```python
from build123d import *

# Parameters (mm, degrees)
BOSS_EXTRUDE1_DEPTH      = 32.5
BOSS_EXTRUDE1_DEPTH_BACK = 20
BOSS_EXTRUDE2_DEPTH      = 30
BOSS_EXTRUDE4_DEPTH      = 25
SKETCH2_W                = 25
SKETCH2_H                = 25
BOSS_EXTRUDE5_DEPTH      = 30
CUT_EXTRUDE1_DEPTH       = 304.293772711
CUT_EXTRUDE1_DEPTH_BACK  = 304.293772711
SKETCH3_R                = 2.5
SKETCH4_W                = 1
SKETCH4_H                = 30
BOSS_EXTRUDE6_DEPTH      = 15
CUT_EXTRUDE2_DEPTH       = 2
CUT_EXTRUDE2_DEPTH_BACK  = 5
SKETCH5_W                = 24.298824304
SKETCH5_H                = 9.719529722
CUT_EXTRUDE3_REACH       = 305.716
SKETCH6_W                = 258.900724606
SKETCH6_H                = 4.300489871
BOSS_EXTRUDE7_DEPTH      = 20


with BuildPart() as part:
    # Sketch1 → Boss-Extrude1 (new, two sides: drawn at the far end of the back side and taken through both)
    with BuildSketch(Plane(origin=(0, 0, 0), x_dir=(1, 0, 0), z_dir=(0, 1, 0)).offset(-BOSS_EXTRUDE1_DEPTH_BACK)):
        with BuildLine():
            ThreePointArc((-255.2, -34.7), (-259.916681078, 0), (-255.2, 34.7))
            ThreePointArc((-255.2, 34.7), (-294.935777018, 0), (-255.2, -34.7))
        make_face()
    extrude(amount=BOSS_EXTRUDE1_DEPTH + BOSS_EXTRUDE1_DEPTH_BACK)



with BuildPart() as body_2:
    # Sketch1<3> → Boss-Extrude2 (new body)
    with BuildSketch(Plane(origin=(0, 0, 0), x_dir=(1, 0, 0), z_dir=(0, 1, 0))):
        with BuildLine():
            ThreePointArc((0, -37.5), (4.396048304, 0), (0, 37.5))
            Line((0, 37.5), (90, 37.5))
            ThreePointArc((90, 37.5), (127.5, 0), (90, -37.5))
            Line((90, -37.5), (0, -37.5))
        make_face()
    extrude(amount=BOSS_EXTRUDE2_DEPTH)


with BuildPart() as part_1:
    add(part.part)

    add(body_2.part)  # Boss-Extrude4 merges body 2
    # Sketch1<5> → Boss-Extrude4 (add)
    with BuildSketch(Plane(origin=(0, 0, 0), x_dir=(1, 0, 0), z_dir=(0, 1, 0))):
        with BuildLine():
            ThreePointArc((3.700724606, -15), (4.396048304, 0), (3.700724606, 15))
            Line((3.700724606, 15), (-259.04839678, 15))
            ThreePointArc((-259.04839678, 15), (-259.916681078, 0), (-259.04839678, -15))
            Line((-259.04839678, -15), (3.700724606, -15))
        make_face()
    extrude(amount=BOSS_EXTRUDE4_DEPTH)

    # Sketch2 → Boss-Extrude5 (add)
    with BuildSketch(Plane.XZ.offset(20)):
        with Locations((-274.43065957, 0)):
            Rectangle(SKETCH2_W, SKETCH2_H)
    extrude(amount=BOSS_EXTRUDE5_DEPTH)

    # Sketch3 → Cut-Extrude1 (cut, two sides: drawn at the far end of the back side and taken through both)
    with BuildSketch(Plane.XY.offset(12.5).offset(-CUT_EXTRUDE1_DEPTH_BACK)):
        with Locations((-279.13065957, -40)):
            Circle(SKETCH3_R)
    extrude(amount=CUT_EXTRUDE1_DEPTH + CUT_EXTRUDE1_DEPTH_BACK, mode=Mode.SUBTRACT)

    # Sketch4 → Boss-Extrude6 (add)
    with BuildSketch(Plane.XZ):
        with Locations((90, 0)):
            Rectangle(SKETCH4_W, SKETCH4_H)
    extrude(amount=BOSS_EXTRUDE6_DEPTH)

    # Sketch5 → Cut-Extrude2 (cut, two sides: drawn at the far end of the back side and taken through both)
    with BuildSketch(Plane(origin=(90.5, 0, 0), x_dir=(0, 0, -1), z_dir=(1, 0, 0)).offset(-CUT_EXTRUDE2_DEPTH_BACK)):
        with Locations((0, -6.741495989)):
            Rectangle(SKETCH5_W, SKETCH5_H)
    extrude(amount=CUT_EXTRUDE2_DEPTH + CUT_EXTRUDE2_DEPTH_BACK, mode=Mode.SUBTRACT)

    # Cut-Extrude3: up to this face of the body (flat: up to its plane)
    cut_extrude3_end = Plane(part_1.part.faces().sort_by_distance((-127.673836087, 12.5, -15))[0])
    # Sketch6 → Cut-Extrude3 (cut, up to the picked face)
    with BuildSketch(Plane.XY.offset(15), mode=Mode.PRIVATE) as cut_extrude3_sk1:
        with Locations((-125.749637697, 2.150244935)):
            Rectangle(SKETCH6_W, SKETCH6_H)
    cut_extrude3_tool1 = split(extrude(cut_extrude3_sk1.sketch, amount=-CUT_EXTRUDE3_REACH, mode=Mode.PRIVATE), bisect_by=cut_extrude3_end, keep=Keep.BOTH, mode=Mode.PRIVATE)
    add(cut_extrude3_tool1.solids().sort_by(Axis((-125.749638, 2.150245, 15), (0, 0, -1)))[0], mode=Mode.SUBTRACT)

    # Sketch7 → Boss-Extrude7 (add)
    with BuildSketch(Plane.XZ.offset(-4.300489871)):
        with BuildLine():
            ThreePointArc((-124.971686685, -5.377242777), (-124.896699141, -5.303300859), (-124.822757223, -5.228313315))
            ThreePointArc((-124.822757223, -5.228313315), (-119.096060376, 0), (-124.822757223, 5.228313315))
            ThreePointArc((-124.822757223, 5.228313315), (-124.896699141, 5.303300859), (-124.971686685, 5.377242777))
            ThreePointArc((-124.971686685, 5.377242777), (-130.2, 11.103939624), (-135.428313315, 5.377242777))
            ThreePointArc((-135.428313315, 5.377242777), (-135.503300859, 5.303300859), (-135.577242777, 5.228313315))
            ThreePointArc((-135.577242777, 5.228313315), (-141.303939624, 0), (-135.577242777, -5.228313315))
            ThreePointArc((-135.577242777, -5.228313315), (-135.503300859, -5.303300859), (-135.428313315, -5.377242777))
            ThreePointArc((-135.428313315, -5.377242777), (-130.2, -11.103939624), (-124.971686685, -5.377242777))
        make_face()
        with BuildLine():
            Line((-132.7, 7.071067812), (-132.7, -7.071067812))
            ThreePointArc((-132.7, -7.071067812), (-130.2, -7.5), (-127.7, -7.071067812))
            Line((-127.7, -7.071067812), (-127.7, 7.071067812))
            ThreePointArc((-127.7, 7.071067812), (-130.2, 7.5), (-132.7, 7.071067812))
        make_face(mode=Mode.SUBTRACT)
    extrude(amount=BOSS_EXTRUDE7_DEPTH)


solid = part_1.part
```
Part model, mm, in its own coordinate system. A direction names the side the tool comes from. Round coordinates to 2 decimals unless told otherwise and drop trailing zeros. Loops run counter-clockwise (first coordinate to the right, second up) from the corner with the lowest first, then second, coordinate; pieces in that order, holes last.
Item 1: Cut at C-C, the plane z = -30. Give the cut face in (x, y).
Item 2: Cut at D-D, the plane x = -159.5. Give the cut face in (y, z).
Item 3: Cut at B-B, the plane y = 9. Give the cut face in (x, z), then the cut area to 3 significant figures.
Item 4: Drop flat-ended pins along their axis: P1, Ø5, axis at x = 24, z = -20, coming from the -Y side; P2, Ø12.5, axis at x = -130, y = 6.5, coming from the +Z side; P3, Ø11.5, axis at y = -1, z = -2, coming from the +X side; P4, Ø11.5, axis at y = -10, z = -1.5, coming from the -X side. Give the stop position or say it passes through.
Item 5: 3-axis set-ups, long thin cutter, end or side, ignore diameter. For faces 1 (the face through (65, 30, -1)), 2 (the face through (-133, -15.7, 0)), 3 (the face through (-127.7, -6, 0)): which of +Z, -Z, +X, -X, +Y, -Y reach the whole face in a straight line?
Item 6: Mould opens along X. For faces 4 (the face through (89.5, -12, 0)), 5 (the face through (90.5, -12, 0)), 6 (the face through (-275, -50, 0)) say: +X half, -X half, draft (parallel to the pull), parting line (faces both ways), or undercut.
Item 7: Cut at A-A, the plane z = 0. State how many separate pieces and enclosed holes the cut face has, then the cut area to 3 significant figures.
Item 8: Drill centre lines: line 1 (X direction, y = -40, z = 0); line 2 (X direction, y = -39.5, z = -7); line 3 (Y direction, x = -76, z = -14.5). Where is each one in solid material? Low to high.
A:
1. outline: (-277.98, -20) - (-256.41, -20) - (-256.41, 32.5) - (-277.98, 32.5) - close; (1.6, 0) - (112.5, 0) - (112.5, 30) - (1.6, 30) - close
2. outline: (4.3, -15) - (25, -15) - (25, 15) - (4.3, 15) - close
3. outline: (-259.05, -15) - (3.7, -15) arc R162.14 cw to (0, -37.5) - (90, -37.5) arc R37.5 ccw to (90, 37.5) - (0, 37.5) arc R162.14 cw to (3.7, 15) - (-259.05, 15) arc R130 cw to (-255.2, 34.7) arc R35.02 ccw (long way) to (-255.2, -34.7) arc R130 cw to start
3. area: 18,700 mm2
4. P1: stops at y = 0
4. P2: stops at z = 15
4. P3: stops at x = 127.5
4. P4: stops at x = -294.94
5. face 1: +Z, -Z, +X, +Y
5. face 2: +Z, -Z, +X, -Y
5. face 3: -Y
6. face 4: undercut
6. face 5: +X half
6. face 6: draft
7. separate pieces: 2
7. enclosed holes: 1
7. area: 12,100 mm2
8. line 1: x = -286.93 to -281.63, -276.63 to -261.93
8. line 2: x = -286.93 to -281.58, -276.68 to -261.93
8. line 3: y = 4.3 to 25
